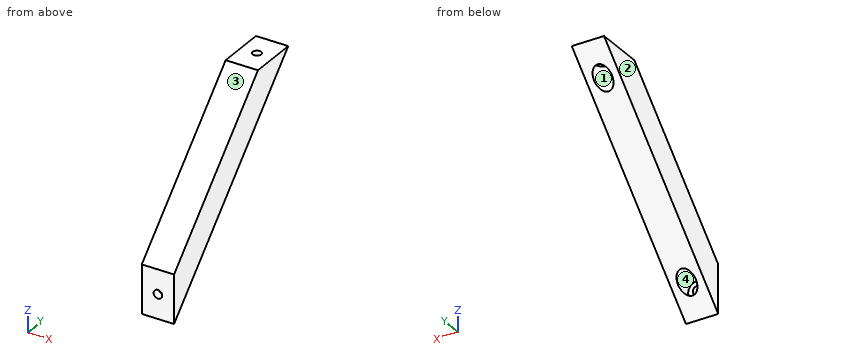
```python
from build123d import *

# Parameters (mm, degrees)
BOSS_EXTRUDE1_DEPTH = 20
SKETCH3_R           = 2.65
CUT_EXTRUDE1_DEPTH  = 114.13708499
SKETCH4_R           = 2.65
CUT_EXTRUDE2_DEPTH  = 114.13708499
SKETCH5_R           = 5.5
CUT_EXTRUDE3_DEPTH  = 109.13708499
SKETCH6_R           = 5.5
CUT_EXTRUDE4_DEPTH  = 109.13708499


with BuildPart() as part:
    # Sketch2 → Boss-Extrude1 (new body)
    with BuildSketch(Plane(origin=(0, 0, 0), x_dir=(0, 0, -1), z_dir=(1, 0, 0))):
        Polygon((0, 0), (-83.13708499, 83.13708499), (-83.13708499, 113.13708499), (30, 0), align=None)
    extrude(amount=BOSS_EXTRUDE1_DEPTH)

    # Sketch3 → Cut-Extrude1 (cut, through all)
    with BuildSketch(Plane.XZ):
        with Locations((10, -15)):
            Circle(SKETCH3_R)
    extrude(amount=-CUT_EXTRUDE1_DEPTH, mode=Mode.SUBTRACT)

    # Sketch4 → Cut-Extrude2 (cut, through all)
    with BuildSketch(Plane.XY.offset(83.13708499)):
        with Locations((10, 98.13708499)):
            Circle(SKETCH4_R)
    extrude(amount=-CUT_EXTRUDE2_DEPTH, mode=Mode.SUBTRACT)

    # Sketch5 → Cut-Extrude3 (cut, through all)
    with BuildSketch(Plane.XY.offset(78.13708499)):
        with Locations((10, 98.13708499)):
            Circle(SKETCH5_R)
    extrude(amount=-CUT_EXTRUDE3_DEPTH, mode=Mode.SUBTRACT)

    # Sketch6 → Cut-Extrude4 (cut, through all)
    with BuildSketch(Plane(origin=(0, 5, 0), x_dir=(-1, 0, 0), z_dir=(0, -1, 0))):
        with Locations((-10, 15)):
            Circle(SKETCH6_R)
    extrude(amount=-CUT_EXTRUDE4_DEPTH, mode=Mode.SUBTRACT)


solid = part.part
```
Source: CAD feature listing. Evaluate the final solid. Frame: model axes, mm. Face numbers are marked on the shaded views. Coordinates: 2 decimals unless noted, no trailing zeros. Write each loop counter-clockwise with the first axis right and the second up, starting at its lowest first coordinate (ties: lowest second). Pieces come first, ordered by that corner, then holes. Notation, with made-up numbers: (78.5, -20.5) - (103.5, -20.5) arc R10 cw to (103.5, -1.5) - close; hole circle Ø2 at (-22, 84.25). An arc over 180 degrees is marked (long way). Answer as a JSON object with one key per item and string values.
Q1. Section query B-B, the plane x = 10. Output: boundary loops of the cut face in (y, z).
Ans:
{"outline": "(0, -30) - (9.5, -20.5) - (5, -20.5) - (5, -17.65) - (0, -17.65) - close; (0, -12.35) - (5, -12.35) - (5, -9.5) - (20.5, -9.5) - (92.64, 62.64) - (92.64, 78.14) - (95.49, 78.14) - (95.49, 83.14) - (83.14, 83.14) - (0, 0) - close; (100.79, 78.14) - (103.64, 78.14) - (103.64, 73.64) - (113.14, 83.14) - (100.79, 83.14) - close"}
Q2. Section query C-C, the plane y = 54. Output: boundary loops of the cut face in (x, z).
Ans:
{"outline": "(0, 24) - (20, 24) - (20, 54) - (0, 54) - close"}
Q3. Draft query along X for the marked faces 1, 2, 3 and 4. Return one class per face: released by +X, released by -X, zero draft, split by the parting line, or undercut.
Ans:
{"face 1": "undercut", "face 2": "released by -X", "face 3": "zero draft", "face 4": "undercut"}
Q4. Section query A-A, the plane z = -15. Output: boundary loops of the cut face in (x, y).
Ans:
{"outline": "(0, 0) - (7.35, 0) - (7.35, 5) - (4.5, 5) - (4.5, 15) - (0, 15) - close; (12.65, 0) - (20, 0) - (20, 15) - (15.5, 15) - (15.5, 5) - (12.65, 5) - close"}
Q5. First-contact query: pin 1 Ø1.5 at (x, z) = (4, 5.5) entering from -Y; pin 2 Ø2 at (x, z) = (8.5, 35.5) entering from -Y; pin 3 Ø6 at (x, y) = (3.5, 46.5) entering from +Z. Flat tips, straight axial feed; report the tip coordinate or a pass-through.
Ans:
{"pin 1": "stops at y = 4.75", "pin 2": "stops at y = 34.5", "pin 3": "stops at z = 49.5"}
Q6. Section query D-D, the plane z = 30.5. Output: boundary loops of the cut face in (x, y).
Ans:
{"outline": "(0, 30.5) - (20, 30.5) - (20, 60.5) - (0, 60.5) - close"}
Q7. Material intervals for line 1 (Z direction, x = 10, y = 2.35); line 2 (Z direction, x = 10, y = 3.55); line 3 (Y direction, x = 10, z = 74.5), sorted ascending. Write a range as [from, to].
Ans:
{"line 1": "z = [-27.65, -17.65], [-12.35, 2.35]", "line 2": "z = [-26.45, -17.65], [-12.35, 3.55]", "line 3": "y = [74.5, 92.64], [103.64, 104.5]"}
